For this review, use the dimensioned drawing (mm, ordinates from the lowest corner) and the shaded views. Coordinates: 2 decimals unless noted, no trailing zeros. Order: outer loops, then holes, each group sorted by start corner. A loop starts at its lowest first (then second) coordinate and runs counter-clockwise, first axis right, second up. Notation, with made-up numbers: M -28.5,25.25 L -23.5,25.25 A23 ccw -23.5,60.25 Z; hole C 84,79 d5. An arc over 180 degrees is marked long. Write each question's results on one line, items separated by ' | '.
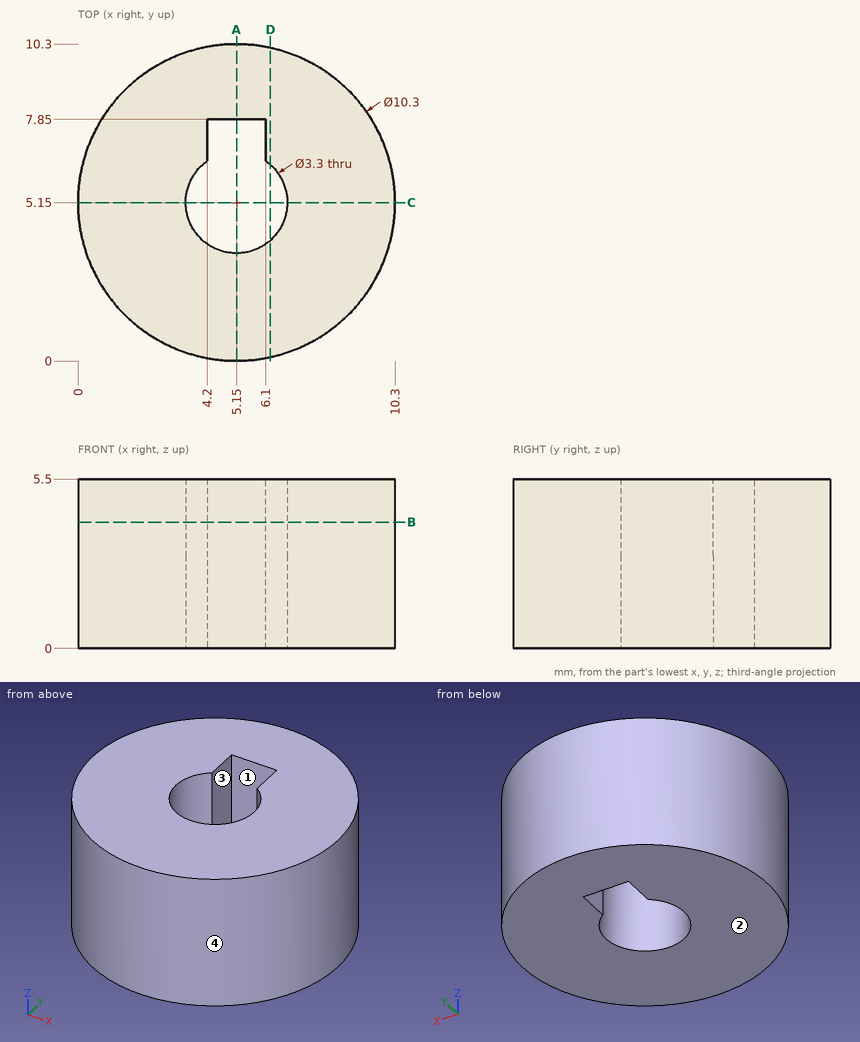
1) To check wall thickness, follow line 1 along Y through (x, z) = (5.25, 2.8); line 2 along X through (y, z) = (5.15, 4.7); line 3 along X through (y, z) = (3.75, 3.95). State the ranges of each line that lie inside material, in increasing order.
Solutions:
line 1: 0 to 3.5, 7.85 to 10.3 | line 2: 0 to 3.5, 6.8 to 10.3 | line 3: 0.19 to 4.28, 6.02 to 10.11
2) For pin 1 (1 mm diameter, centred on x = 6.5, z = 4, fed in from +Y); pin 2 (1 mm diameter, centred on x = 5.5, z = 2.5, fed in from +Y); pin 3 (1.5 mm diameter, centred on y = 7, z = 3.5, fed in from +X); pin 4 (1.5 mm diameter, centred on y = 7, z = 1.5, fed in from -X), all flat-tipped, find the tip position at first contact; note any pin that passes through.
Solutions:
pin 1: y = 10.23 | pin 2: y = 10.3 | pin 3: x = 10.18 | pin 4: x = 0.12
3) Take a section at A-A on x = 5.15. State the section outline as (y, z) points.
Solutions:
outline: M 0,0 L 3.5,0 L 3.5,5.5 L 0,5.5 Z; M 7.85,0 L 10.3,0 L 10.3,5.5 L 7.85,5.5 Z
4) Take a section at D-D on x = 6.25. State the section outline as (y, z) points, plus the area to 3 significant figures.
Solutions:
outline: M 0.12,0 L 3.92,0 L 3.92,5.5 L 0.12,5.5 Z; M 6.38,0 L 10.18,0 L 10.18,5.5 L 6.38,5.5 Z | area: 41.8 mm2
5) The part is to be moulded in two halves that separate along Y. For the marked faces 1, 2, 3 and 4, say which applies: pulls with the +Y half, pulls with the -Y half, needs draft (parallel to the pull), parting line crosses it, or undercut.
Solutions:
face 1: undercut | face 2: needs draft | face 3: undercut | face 4: parting line crosses it
6) Take a section at C-C on y = 5.15. State the section outline as (x, z) points.
Solutions:
outline: M 0,0 L 3.5,0 L 3.5,5.5 L 0,5.5 Z; M 6.8,0 L 10.3,0 L 10.3,5.5 L 6.8,5.5 Z
7) Take a section at B-B on z = 4.1. State the section outline as (x, y) points.
Solutions:
outline: C 5.15,5.15 d10.3; hole M 4.2,6.5 A1.65 ccw long 6.1,6.5 L 6.1,7.85 L 4.2,7.85 Z
